from build123d import *

# Parameters (mm, degrees)
PAD001_DEPTH = 15
SKETCH002_W  = 50
SKETCH002_H  = 80
PAD002_DEPTH = 20
SKETCH003_W  = 10
SKETCH003_H  = 80
PAD003_DEPTH = 10


with BuildPart() as part:
    # Sketch001 → Pad001 (new body, symmetric)
    with BuildSketch(Plane(origin=(0, 0, 0), x_dir=(0, -1, 0), z_dir=(-1, 0, 0))):
        Polygon((0, 20), (50, 20), (-10.621778, 55), (-60.621778, 55), align=None)
    extrude(amount=PAD001_DEPTH, both=True)

    # Sketch002 → Pad002 (new body)
    with BuildSketch(Plane(origin=(0, 0, 55), x_dir=(0, 1, 0), z_dir=(0, 0, 1))):
        with Locations((35.621778, 0)):
            Rectangle(SKETCH002_W, SKETCH002_H)
    extrude(amount=PAD002_DEPTH)

    # Sketch003 → Pad003 (new body)
    with BuildSketch(Plane(origin=(0, 0, 75), x_dir=(0, 1, 0), z_dir=(0, 0, 1))):
        with Locations((15.621778, 0)):
            Rectangle(SKETCH003_W, SKETCH003_H)
    extrude(amount=PAD003_DEPTH)


solid = part.part
Could you check a few things on this model? Use its own coordinates, in mm. A direction names the side the tool comes from. Round coordinates to 2 decimals unless told otherwise and drop trailing zeros. Loops run counter-clockwise (first coordinate to the right, second up) from the corner with the lowest first, then second, coordinate; pieces in that order, holes last. Notation, with made-up numbers: (42.5, 10.5) - (86.5, 10.5) arc R14 ccw to (86.5, 31.5) - close; hole circle Ø10 at (26.25, 63.5). An arc over 180 degrees is marked (long way). Write item = value, one per line.
1) I'm going to push flat-ended pins straight in: P1, Ø9, axis at x = 17.5, z = 72.5, coming from the -Y side; P2, Ø20, axis at x = -29.5, y = 44.5, coming from the -Z side; P3, Ø8, axis at x = -12.5, z = 80.5, coming from the +Y side. Where does each tip first touch, or does it pass through?
Computed:
P1 = 10.62
P2 = 55
P3 = 20.62
2) Imagine slicing it at D-D (x = -25.5). Please give me the cut outline in (y, z), and give its area (3 significant figures).
Computed:
outline = (10.62, 55) - (60.62, 55) - (60.62, 75) - (20.62, 75) - (20.62, 85) - (10.62, 85) - close
area = 1,100 mm2
3) On a 3-axis mill with a long thin cutter (end or side, diameter ignored), from which of +Z, -Z, +X, -X, +Y, -Y can I reach the whole of each face in a straight line? I mean faces 1 (the flat face through (-15, 6, 38)), 2 (the flat face through (-0.21, 30.735, 37.745)), 3 (the flat face through (1, 10.622, 70)), 4 (the flat face through (-1, 40, 75)), 5 (the flat face through (15, 6, 38)). Say none if no direction works.
Computed:
face_1 = -Z, -X, +Y, -Y
face_2 = -Z, +X, -X, +Y
face_3 = +Z, +X, -X, -Y
face_4 = +Z, +X, -X, +Y
face_5 = -Z, +X, +Y, -Y
4) I need wall thicknesses on line 1 along X through (y, z) = (24.5, 48); line 2 along Y through (x, z) = (-31, 76); line 3 along Z through (x, y) = (24.5, 13.5). Which ranges of each line are inside material? Lowest first, please. Write a range as from..to.
Computed:
line_1 = -15..15
line_2 = 10.62..20.62
line_3 = 55..85
5) Imagine slicing it at B-B (x = -0.5). Please give me the cut outline in (y, z), and give its area (3 significant figures).
Computed:
outline = (-50, 20) - (0, 20) - (60.62, 55) - (60.62, 75) - (20.62, 75) - (20.62, 85) - (10.62, 85) - (10.62, 55) - close
area = 2,850 mm2
6) Imagine slicing it at C-C (z = 62.5). Please give me the cut outline in (x, y).
Computed:
outline = (-40, 10.62) - (40, 10.62) - (40, 60.62) - (-40, 60.62) - close
7) Imagine slicing it at A-A (y = 39). Please give me the cut outline in (x, z), and give its area (3 significant figures).
Computed:
outline = (-40, 55) - (-15, 55) - (-15, 42.52) - (15, 42.52) - (15, 55) - (40, 55) - (40, 75) - (-40, 75) - close
area = 1,970 mm2
